Input: dimensioned drawing with shaded views. Units: mm. Origin: part minimum x, y, z. A direction names the side the tool comes from. Coordinates: 2 decimals unless noted, no trailing zeros. Order: outer loops, then holes, each group sorted by start corner. A loop starts at its lowest first (then second) coordinate and runs counter-clockwise, first axis right, second up. Notation, with made-up numbers: (48.5, 15.25) -> (69.5, 15.25) arc R12 ccw to (69.5, 35.25) -> close; hole circle Ø5 at (78.5, 59.25). An arc over 180 degrees is marked (long way). Write item = value, one per line. Start each with the question number.
Item 1: Ray query, line 1 along Y through (x, z) = (4.5, 72.5); line 2 along Z through (x, y) = (32.5, 20). Return the intervals inside material, ascending. Write a range as [from, to].
Item 2: Set-up query: the marked faces 1 and 2. Return all of +Z, -Z, +X, -X, +Y, -Y with unobstructed straight access to the full face (end or side cutting, diameter ignored); none if empty.
Item 3: Section query A-A (y = 4). Output: boundary loops of the cut face in (x, z).
Item 4: Contact query for flat-ended pins moving along their axis: pin 1 (2 mm diameter, centred on x = 26, y = 24.5, fed in from -Z); pin 2 (2.5 mm diameter, centred on x = 1, y = 46, fed in from -Z); pin 3 (8 mm diameter, centred on x = 14.5, y = 8.5, fed in from -Z); pin 4 (3.5 mm diameter, centred on x = 1, y = 46.5, fed in from +Z). Output: stop coordinate, or through.
Item 5: Section query C-C (z = 91.5). Output: boundary loops of the cut face in (x, y), then the cut area to 3 significant figures.
Item 6: Section query B-B (x = 19). Output: boundary loops of the cut face in (y, z), then the cut area to 3 significant figures.
Item 7: Section query D-D (y = 42.5). Output: boundary loops of the cut face in (x, z).
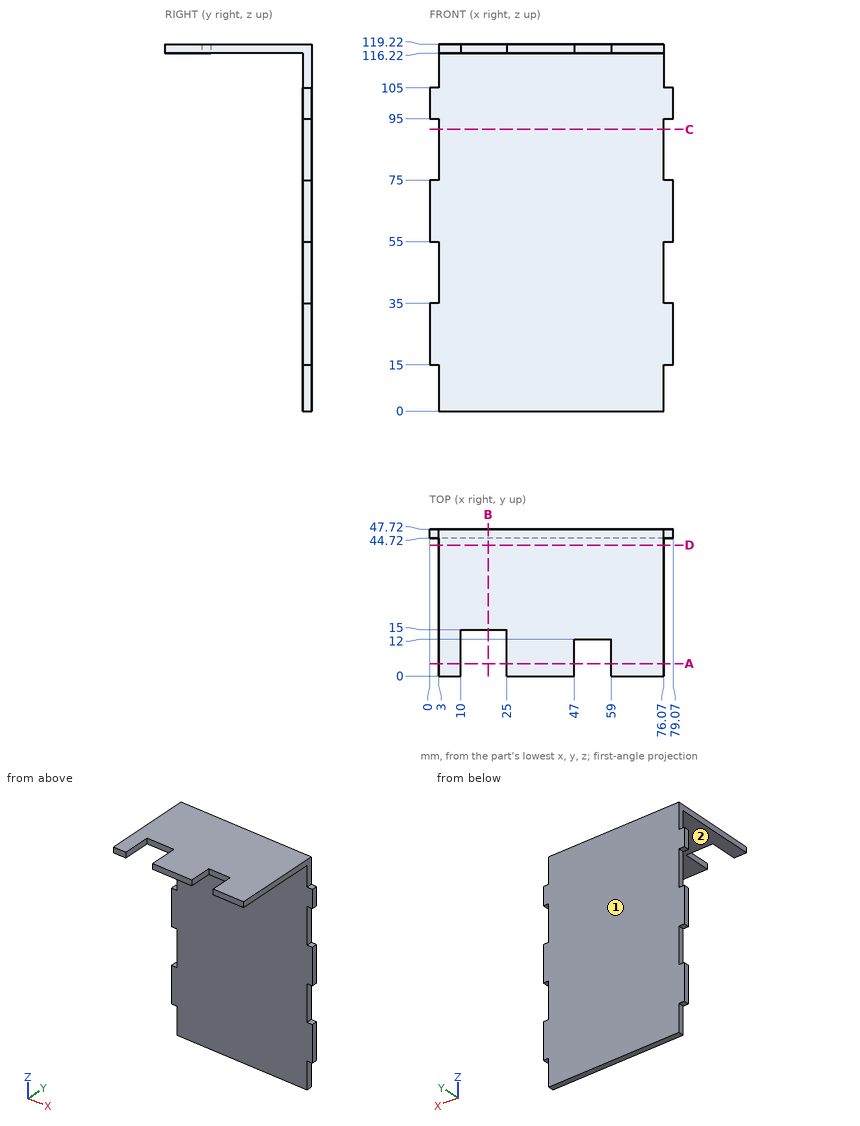
Computed:
q1.line_1 = [44.72, 47.72]
q1.line_2 = [116.22, 119.22]
q2.face_1 = +Z, -Z, +X, -X, +Y
q2.face_2 = -Z, +X, -X, -Y
q3.outline = (3, 116.22) -> (10, 116.22) -> (10, 119.22) -> (3, 119.22) -> close; (25, 116.22) -> (47, 116.22) -> (47, 119.22) -> (25, 119.22) -> close; (59, 116.22) -> (76.07, 116.22) -> (76.07, 119.22) -> (59, 119.22) -> close
q4.pin_1 = 116.22
q4.pin_2 = 15
q4.pin_3 = through
q4.pin_4 = 105
q5.outline = (3, 44.72) -> (76.07, 44.72) -> (76.07, 47.72) -> (3, 47.72) -> close
q5.area = 219 mm^2
q6.outline = (15, 116.22) -> (44.72, 116.22) -> (44.72, 0) -> (47.72, 0) -> (47.72, 119.22) -> (15, 119.22) -> close
q6.area = 447 mm^2
q7.outline = (3, 116.22) -> (76.07, 116.22) -> (76.07, 119.22) -> (3, 119.22) -> close
